Geometry: final body of the model. Coordinates: model frame, mm. A direction names the side the tool comes from. Round coordinates to 2 decimals unless told otherwise and drop trailing zeros. Loops run counter-clockwise (first coordinate to the right, second up) from the corner with the lowest first, then second, coordinate; pieces in that order, holes last. Notation, with made-up numbers: (48.5, -30) -> (83.5, -30) arc R14 ccw to (83.5, -12) -> close; hole circle Ø8 at (37.25, 11). An arc over 180 degrees is marked (long way). Answer in a Markdown table with one row per item.
```python
from build123d import *

# Parameters (mm, degrees)
BOSS_EXTRUDE1_DEPTH = 127


with BuildPart() as part:
    # Sketch1 → Boss-Extrude1 (new body)
    with BuildSketch(Plane(origin=(0, 0, 0), x_dir=(0, 0, -1), z_dir=(1, 0, 0))):
        with BuildLine():
            Line((23.1902, 19.174899798), (23.1902, 17.0561))
            ThreePointArc((23.1902, 17.0561), (24.2951, 15.9512), (25.4, 17.0561))
            Line((25.4, 17.0561), (25.4, 23.2918))
            ThreePointArc((25.4, 23.2918), (24.782522516, 24.782522516), (23.2918, 25.4))
            Line((23.2918, 25.4), (17.0561, 25.4))
            ThreePointArc((17.0561, 25.4), (15.9512, 24.2951), (17.0561, 23.1902))
            Line((17.0561, 23.1902), (19.174899798, 23.1902))
            ThreePointArc((19.174899798, 23.1902), (20.113561403, 22.563006367), (19.893320288, 21.45577951))
            Line((19.893320288, 21.45577951), (16.58464389, 18.147103113))
            ThreePointArc((16.58464389, 18.147103113), (15.554599758, 17.458849627), (14.33957986, 17.217167143))
            Line((14.33957986, 17.217167143), (11.06042014, 17.217167143))
            ThreePointArc((11.06042014, 17.217167143), (9.845400242, 17.458849627), (8.81535611, 18.147103113))
            Line((8.81535611, 18.147103113), (5.506679712, 21.45577951))
            ThreePointArc((5.506679712, 21.45577951), (5.286438597, 22.563006367), (6.225100202, 23.1902))
            Line((6.225100202, 23.1902), (8.3439, 23.1902))
            ThreePointArc((8.3439, 23.1902), (9.4488, 24.2951), (8.3439, 25.4))
            Line((8.3439, 25.4), (-8.3439, 25.4))
            ThreePointArc((-8.3439, 25.4), (-9.4488, 24.2951), (-8.3439, 23.1902))
            Line((-8.3439, 23.1902), (-6.225100202, 23.1902))
            ThreePointArc((-6.225100202, 23.1902), (-5.286438597, 22.563006367), (-5.506679712, 21.45577951))
            Line((-5.506679712, 21.45577951), (-8.81535611, 18.147103113))
            ThreePointArc((-8.81535611, 18.147103113), (-9.845400242, 17.458849627), (-11.06042014, 17.217167143))
            Line((-11.06042014, 17.217167143), (-14.33957986, 17.217167143))
            ThreePointArc((-14.33957986, 17.217167143), (-15.554599758, 17.458849627), (-16.58464389, 18.147103113))
            Line((-16.58464389, 18.147103113), (-19.893320288, 21.45577951))
            ThreePointArc((-19.893320288, 21.45577951), (-20.113561403, 22.563006367), (-19.174899798, 23.1902))
            Line((-19.174899798, 23.1902), (-17.0561, 23.1902))
            ThreePointArc((-17.0561, 23.1902), (-15.9512, 24.2951), (-17.0561, 25.4))
            Line((-17.0561, 25.4), (-23.2918, 25.4))
            ThreePointArc((-23.2918, 25.4), (-24.782522516, 24.782522516), (-25.4, 23.2918))
            Line((-25.4, 23.2918), (-25.4, 17.0561))
            ThreePointArc((-25.4, 17.0561), (-24.2951, 15.9512), (-23.1902, 17.0561))
            Line((-23.1902, 17.0561), (-23.1902, 19.174899798))
            ThreePointArc((-23.1902, 19.174899798), (-22.563006367, 20.113561403), (-21.45577951, 19.893320288))
            Line((-21.45577951, 19.893320288), (-18.147103113, 16.58464389))
            ThreePointArc((-18.147103113, 16.58464389), (-17.458849627, 15.554599758), (-17.217167143, 14.33957986))
            Line((-17.217167143, 14.33957986), (-17.217167143, 11.06042014))
            ThreePointArc((-17.217167143, 11.06042014), (-17.458849627, 9.845400242), (-18.147103113, 8.81535611))
            Line((-18.147103113, 8.81535611), (-21.45577951, 5.506679712))
            ThreePointArc((-21.45577951, 5.506679712), (-22.563006367, 5.286438597), (-23.1902, 6.225100202))
            Line((-23.1902, 6.225100202), (-23.1902, 8.3439))
            ThreePointArc((-23.1902, 8.3439), (-24.2951, 9.4488), (-25.4, 8.3439))
            Line((-25.4, 8.3439), (-25.4, -8.3439))
            ThreePointArc((-25.4, -8.3439), (-24.2951, -9.4488), (-23.1902, -8.3439))
            Line((-23.1902, -8.3439), (-23.1902, -6.225100202))
            ThreePointArc((-23.1902, -6.225100202), (-22.563006367, -5.286438597), (-21.45577951, -5.506679712))
            Line((-21.45577951, -5.506679712), (-18.147103113, -8.81535611))
            ThreePointArc((-18.147103113, -8.81535611), (-17.458849627, -9.845400242), (-17.217167143, -11.06042014))
            Line((-17.217167143, -11.06042014), (-17.217167143, -14.33957986))
            ThreePointArc((-17.217167143, -14.33957986), (-17.458849627, -15.554599758), (-18.147103113, -16.58464389))
            Line((-18.147103113, -16.58464389), (-21.45577951, -19.893320288))
            ThreePointArc((-21.45577951, -19.893320288), (-22.563006367, -20.113561403), (-23.1902, -19.174899798))
            Line((-23.1902, -19.174899798), (-23.1902, -17.0561))
            ThreePointArc((-23.1902, -17.0561), (-24.2951, -15.9512), (-25.4, -17.0561))
            Line((-25.4, -17.0561), (-25.4, -23.2918))
            ThreePointArc((-25.4, -23.2918), (-24.782522516, -24.782522516), (-23.2918, -25.4))
            Line((-23.2918, -25.4), (-17.0561, -25.4))
            ThreePointArc((-17.0561, -25.4), (-15.9512, -24.2951), (-17.0561, -23.1902))
            Line((-17.0561, -23.1902), (-19.174899798, -23.1902))
            ThreePointArc((-19.174899798, -23.1902), (-20.113561403, -22.563006367), (-19.893320288, -21.45577951))
            Line((-19.893320288, -21.45577951), (-16.58464389, -18.147103113))
            ThreePointArc((-16.58464389, -18.147103113), (-15.554599758, -17.458849627), (-14.33957986, -17.217167143))
            Line((-14.33957986, -17.217167143), (-11.06042014, -17.217167143))
            ThreePointArc((-11.06042014, -17.217167143), (-9.845400242, -17.458849627), (-8.81535611, -18.147103113))
            Line((-8.81535611, -18.147103113), (-5.506679712, -21.45577951))
            ThreePointArc((-5.506679712, -21.45577951), (-5.286438597, -22.563006367), (-6.225100202, -23.1902))
            Line((-6.225100202, -23.1902), (-8.3439, -23.1902))
            ThreePointArc((-8.3439, -23.1902), (-9.4488, -24.2951), (-8.3439, -25.4))
            Line((-8.3439, -25.4), (8.3439, -25.4))
            ThreePointArc((8.3439, -25.4), (9.4488, -24.2951), (8.3439, -23.1902))
            Line((8.3439, -23.1902), (6.225100202, -23.1902))
            ThreePointArc((6.225100202, -23.1902), (5.286438597, -22.563006367), (5.506679712, -21.45577951))
            Line((5.506679712, -21.45577951), (8.81535611, -18.147103113))
            ThreePointArc((8.81535611, -18.147103113), (9.845400242, -17.458849627), (11.06042014, -17.217167143))
            Line((11.06042014, -17.217167143), (14.33957986, -17.217167143))
            ThreePointArc((14.33957986, -17.217167143), (15.554599758, -17.458849627), (16.58464389, -18.147103113))
            Line((16.58464389, -18.147103113), (19.893320288, -21.45577951))
            ThreePointArc((19.893320288, -21.45577951), (20.113561403, -22.563006367), (19.174899798, -23.1902))
            Line((19.174899798, -23.1902), (17.0561, -23.1902))
            ThreePointArc((17.0561, -23.1902), (15.9512, -24.2951), (17.0561, -25.4))
            Line((17.0561, -25.4), (23.2918, -25.4))
            ThreePointArc((23.2918, -25.4), (24.782522516, -24.782522516), (25.4, -23.2918))
            Line((25.4, -23.2918), (25.4, -17.0561))
            ThreePointArc((25.4, -17.0561), (24.2951, -15.9512), (23.1902, -17.0561))
            Line((23.1902, -17.0561), (23.1902, -19.174899798))
            ThreePointArc((23.1902, -19.174899798), (22.563006367, -20.113561403), (21.45577951, -19.893320288))
            Line((21.45577951, -19.893320288), (18.147103113, -16.58464389))
            ThreePointArc((18.147103113, -16.58464389), (17.458849627, -15.554599758), (17.217167143, -14.33957986))
            Line((17.217167143, -14.33957986), (17.217167143, -11.06042014))
            ThreePointArc((17.217167143, -11.06042014), (17.458849627, -9.845400242), (18.147103113, -8.81535611))
            Line((18.147103113, -8.81535611), (21.45577951, -5.506679712))
            ThreePointArc((21.45577951, -5.506679712), (22.563006367, -5.286438597), (23.1902, -6.225100202))
            Line((23.1902, -6.225100202), (23.1902, -8.3439))
            ThreePointArc((23.1902, -8.3439), (24.2951, -9.4488), (25.4, -8.3439))
            Line((25.4, -8.3439), (25.4, 8.3439))
            ThreePointArc((25.4, 8.3439), (24.2951, 9.4488), (23.1902, 8.3439))
            Line((23.1902, 8.3439), (23.1902, 6.225100202))
            ThreePointArc((23.1902, 6.225100202), (22.563006367, 5.286438597), (21.45577951, 5.506679712))
            Line((21.45577951, 5.506679712), (18.147103113, 8.81535611))
            ThreePointArc((18.147103113, 8.81535611), (17.458849627, 9.845400242), (17.217167143, 11.06042014))
            Line((17.217167143, 11.06042014), (17.217167143, 14.33957986))
            ThreePointArc((17.217167143, 14.33957986), (17.458849627, 15.554599758), (18.147103113, 16.58464389))
            Line((18.147103113, 16.58464389), (21.45577951, 19.893320288))
            ThreePointArc((21.45577951, 19.893320288), (22.563006367, 20.113561403), (23.1902, 19.174899798))
        make_face()
        with BuildLine():
            Line((8.182832857, -10.392632857), (8.182832857, -14.739168105))
            ThreePointArc((8.182832857, -14.739168105), (8.014621848, -15.584821954), (7.535597422, -16.30173267))
            Line((7.535597422, -16.30173267), (2.058651438, -21.778678654))
            ThreePointArc((2.058651438, -21.778678654), (0, -22.6314), (-2.058651438, -21.778678654))
            Line((-2.058651438, -21.778678654), (-7.535597422, -16.30173267))
            ThreePointArc((-7.535597422, -16.30173267), (-8.014621848, -15.584821954), (-8.182832857, -14.739168105))
            Line((-8.182832857, -14.739168105), (-8.182832857, -10.392632857))
            ThreePointArc((-8.182832857, -10.392632857), (-8.830068292, -8.830068292), (-10.392632857, -8.182832857))
            Line((-10.392632857, -8.182832857), (-14.739168105, -8.182832857))
            ThreePointArc((-14.739168105, -8.182832857), (-15.584821954, -8.014621848), (-16.30173267, -7.535597422))
            Line((-16.30173267, -7.535597422), (-21.778678654, -2.058651438))
            ThreePointArc((-21.778678654, -2.058651438), (-22.6314, 0), (-21.778678654, 2.058651438))
            Line((-21.778678654, 2.058651438), (-16.30173267, 7.535597422))
            ThreePointArc((-16.30173267, 7.535597422), (-15.584821954, 8.014621848), (-14.739168105, 8.182832857))
            Line((-14.739168105, 8.182832857), (-10.392632857, 8.182832857))
            ThreePointArc((-10.392632857, 8.182832857), (-8.830068292, 8.830068292), (-8.182832857, 10.392632857))
            Line((-8.182832857, 10.392632857), (-8.182832857, 14.739168105))
            ThreePointArc((-8.182832857, 14.739168105), (-8.014621848, 15.584821954), (-7.535597422, 16.30173267))
            Line((-7.535597422, 16.30173267), (-2.058651438, 21.778678654))
            ThreePointArc((-2.058651438, 21.778678654), (0, 22.6314), (2.058651438, 21.778678654))
            Line((2.058651438, 21.778678654), (7.535597422, 16.30173267))
            ThreePointArc((7.535597422, 16.30173267), (8.014621848, 15.584821954), (8.182832857, 14.739168105))
            Line((8.182832857, 14.739168105), (8.182832857, 10.392632857))
            ThreePointArc((8.182832857, 10.392632857), (8.830068292, 8.830068292), (10.392632857, 8.182832857))
            Line((10.392632857, 8.182832857), (14.739168105, 8.182832857))
            ThreePointArc((14.739168105, 8.182832857), (15.584821954, 8.014621848), (16.30173267, 7.535597422))
            Line((16.30173267, 7.535597422), (21.778678654, 2.058651438))
            ThreePointArc((21.778678654, 2.058651438), (22.6314, 0), (21.778678654, -2.058651438))
            Line((21.778678654, -2.058651438), (16.30173267, -7.535597422))
            ThreePointArc((16.30173267, -7.535597422), (15.584821954, -8.014621848), (14.739168105, -8.182832857))
            Line((14.739168105, -8.182832857), (10.392632857, -8.182832857))
            ThreePointArc((10.392632857, -8.182832857), (8.830068292, -8.830068292), (8.182832857, -10.392632857))
        make_face(mode=Mode.SUBTRACT)
    extrude(amount=-BOSS_EXTRUDE1_DEPTH)


solid = part.part
```
Item 1: Pin query (flat end, axial travel): pin 1 Ø2 at (x, y) = (-81, 13.5) entering from +Z; pin 2 Ø3.5 at (x, z) = (-44, 12.5) entering from -Y; pin 3 Ø6 at (x, z) = (-36.5, 12) entering from -Y. Return the tip coordinate at first contact, or that it passes through.
Answer:
| item | result |
|---|---|
| pin 1 | stops at z = 17.22 |
| pin 2 | stops at y = -17.23 |
| pin 3 | stops at y = -25.18 |
Item 2: Line query: probe 1 along Y at (x, z) = (-36, -17.5); probe 2 along Y at (x, z) = (-35.5, 23.5); probe 3 along Y at (x, z) = (-66, -23). Output: solid intervals per line, ascending. Write a range as [from, to].
Answer:
| item | result |
|---|---|
| probe 1 | y = [-25.4, -23.19], [-19.06, -15.65], [-9.75, -6.34], [6.34, 9.75], [15.65, 19.06], [23.19, 25.4] |
| probe 2 | y = [-25.39, -16.29], [-9.11, 9.11], [16.29, 25.39] |
| probe 3 | y = [-25.4, -19.77], [-5.63, 5.63], [19.77, 25.4] |
Item 3: Cut plane A-A (z = -3.5). Output: boundary loops of the cut face in (x, y), then the cut area to 3 significant figures.
Answer:
| item | result |
|---|---|
| outline | (-127, -25.4) -> (0, -25.4) -> (0, -20.34) -> (-127, -20.34) -> close; (-127, 20.34) -> (0, 20.34) -> (0, 25.4) -> (-127, 25.4) -> close |
| area | 1,290 mm² |
Item 4: Reachability of faces 5 (the face through (-63, 0, -25.4)), 6 (the face through (-62.61, 19.08, -4.76)), 7 (the face through (-63, 17.217, 13)) from +Z, -Z, +X, -X, +Y, -Y: full face, straight path, thin tool, end or side. Return the list, or none.
Answer:
| item | result |
|---|---|
| face 5 | -Z, +X, -X, +Y, -Y |
| face 6 | +X, -X |
| face 7 | +X, -X, +Y |
Item 5: Draft query along Z for faces 1 (the face through (-63, 25.4, 20)), 2 (the face through (-62.61, 4.84, -19)), 3 (the face through (-63, -20, 25.4)), 4 (the face through (-63, 13, -17.217)). Return one class per face: pulls with the +Z half, pulls with the -Z half, needs draft (parallel to the pull), parting line crosses it, or undercut.
Answer:
| item | result |
|---|---|
| face 1 | needs draft |
| face 2 | undercut |
| face 3 | pulls with the +Z half |
| face 4 | pulls with the -Z half |
